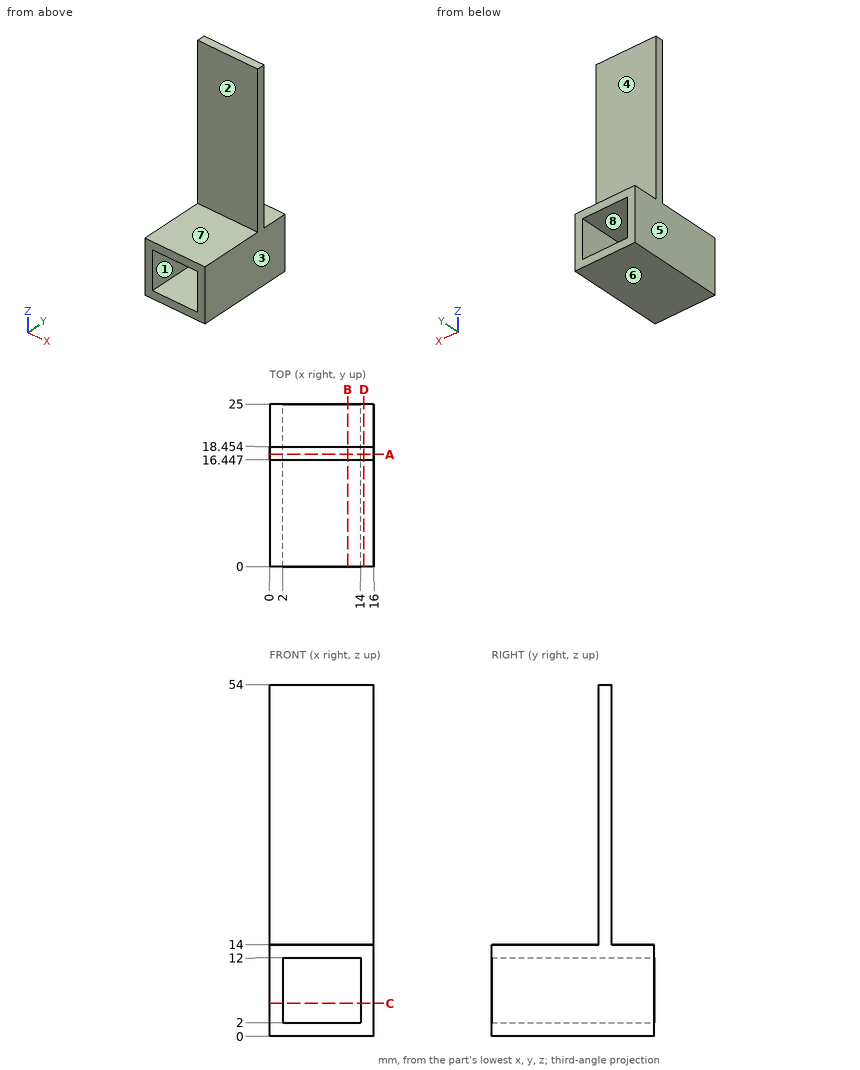
Answer from the drawing. Dimensions are ordinates in mm from the lowest x, y and z of the part. A direction names the side the tool comes from. Round coordinates to 2 decimals unless told otherwise and drop trailing zeros. Loops run counter-clockwise (first coordinate to the right, second up) from the corner with the lowest first, then second, coordinate; pieces in that order, holes last. Notation, with made-up numbers: (76.5, 23.5) - (90.5, 23.5) arc R33 cw to (90.5, 52.5) - close; hole circle Ø2 at (56, 17). An arc over 180 degrees is marked (long way). Return JSON: item names as keys, results as strings. Group by question number.
1. The part is cut by section D-D on x = 14.5. Determine the outline of the cut face in (y, z) (1 decimal).
2. The part is cut by section A-A on y = 17.25. Determine the outline of the cut face in (x, z).
3. The part is cut by section B-B on x = 12. Determine the outline of the cut face in (y, z) (1 decimal).
4. Consider probe 1 along Z at (x, y) = (9.5, 7.25); probe 2 along X at (y, z) = (6.5, 3.5); probe 3 along Y at (x, z) = (10, 35.5) (1 decimal). Determine where each line is inside the solid, lowest interval first.
5. The mould has two halves that part along X. Classify the marked faces 1, 2 and 3: pulls with the +X half, pulls with the -X half, needs draft (parallel to the pull), parting line crosses it, or undercut.
6. Each of these flat-tipped pins is pushed along its axis until it touches: P1, Ø5, axis at x = 9, y = 22.5, coming from the +Z side; P2, Ø4, axis at x = 3, z = 23.5, coming from the +Y side. Where does it stop, or does it pass through?
7. Which of the six approach directions +Z, -Z, +X, -X, +Y, -Y give full straight-line access (tool end or side, diameter ignored) to the marked faces 4, 5, 6, 7 and 8?
8. The part is cut by section C-C on z = 5. Determine the outline of the cut face in (x, y).
Resolved:
{
 "1": {"outline": "(0, 0) - (25, 0) - (25, 14) - (18.5, 14) - (18.5, 54) - (16.4, 54) - (16.4, 14) - (0, 14) - close"},
 "2": {"outline": "(0, 0) - (16, 0) - (16, 54) - (0, 54) - close; hole (2, 2) - (14, 2) - (14, 12) - (2, 12) - close"},
 "3": {"outline": "(0, 0) - (25, 0) - (25, 2) - (0, 2) - close; (0, 12) - (25, 12) - (25, 14) - (18.5, 14) - (18.5, 54) - (16.4, 54) - (16.4, 14) - (0, 14) - close"},
 "4": {"probe 1": "z = 0 to 2, 12 to 14", "probe 2": "x = 0 to 2, 14 to 16", "probe 3": "y = 16.4 to 18.5"},
 "5": {"face 1": "undercut", "face 2": "needs draft", "face 3": "pulls with the +X half"},
 "6": {"P1": "stops at z = 14", "P2": "stops at y = 18.45"},
 "7": {"face 4": "+Z, +X, -X, +Y", "face 5": "+Z, -Z, -X, +Y, -Y", "face 6": "-Z, +X, -X, +Y, -Y", "face 7": "+Z, +X, -X, -Y", "face 8": "+Y, -Y"},
 "8": {"outline": "(0, 0) - (2, 0) - (2, 25) - (0, 25) - close; (14, 0) - (16, 0) - (16, 25) - (14, 25) - close"}
}
